from build123d import *

# Parameters (mm, degrees)
SKETCH1_W                                           = 60
SKETCH1_H                                           = 35
BOSS_EXTRUDE1_DEPTH                                 = 3
BOSS_EXTRUDE2_DEPTH                                 = 60
CUT_EXTRUDE4_DEPTH                                  = 49.961719741
CUT_EXTRUDE4_DEPTH_BACK                             = 49.961719741
SKETCH9_W                                           = 15
SKETCH9_H                                           = 12
CSK_FOR_M3_COUNTERSUNK_FLAT_HEAD_SCREW1_D           = 3.4
CSK_FOR_M3_COUNTERSUNK_FLAT_HEAD_SCREW1_DEPTH       = 3
CSK_FOR_M3_COUNTERSUNK_FLAT_HEAD_SCREW1_CSINK_D     = 6.3
CSK_FOR_M3_COUNTERSUNK_FLAT_HEAD_SCREW1_CSINK_ANGLE = 90
CSK_FOR_M3_COUNTERSUNK_FLAT_HEAD_SCREW1_TIP         = 1.021463052


with BuildPart() as part:
    # Sketch1 → Boss-Extrude1 (new body)
    with BuildSketch(Plane.XY):
        Rectangle(SKETCH1_W, SKETCH1_H)
    extrude(amount=BOSS_EXTRUDE1_DEPTH)

    # Sketch5 → Boss-Extrude2 (add)
    with BuildSketch(Plane(origin=(30, 0, 0), x_dir=(0, 0, -1), z_dir=(1, 0, 0))):
        with BuildLine():
            Line((-5.479055467, 14.545576741), (-4.958110934, 11.591153482))
            ThreePointArc((-4.958110934, 11.591153482), (-8.05212086, 23.138155725), (-3, 12.303847577))
            Line((-3, 12.303847577), (-3, 17.5))
            ThreePointArc((-3, 17.5), (-8.298133329, 19.428362829), (-5.479055467, 14.545576741))
        make_face()
    extrude(amount=-BOSS_EXTRUDE2_DEPTH)

    # Sketch9 → Cut-Extrude4 (cut, two sides: drawn at the far end of the back side and taken through both)
    with BuildSketch(Plane(origin=(-12, 0, 3), x_dir=(-1, 0, 0), z_dir=(0, 0, -1)).offset(-CUT_EXTRUDE4_DEPTH_BACK)):
        with Locations((-19.5, 17.5)):
            Rectangle(SKETCH9_W, SKETCH9_H)
        with Locations((10.5, 17.5)):
            Rectangle(SKETCH9_W, SKETCH9_H)
    extrude(amount=CUT_EXTRUDE4_DEPTH + CUT_EXTRUDE4_DEPTH_BACK, mode=Mode.SUBTRACT)

    # CSK for M3 Countersunk Flat Head Screw1
    with Locations(Plane(origin=(0, 0, 0), x_dir=(1, 0, 0), z_dir=(0, 0, -1))):
        with Locations((0, -4.5), (-15, 9.5), (15, 9.5)):
            CounterSinkHole(CSK_FOR_M3_COUNTERSUNK_FLAT_HEAD_SCREW1_D / 2, CSK_FOR_M3_COUNTERSUNK_FLAT_HEAD_SCREW1_CSINK_D / 2, depth=CSK_FOR_M3_COUNTERSUNK_FLAT_HEAD_SCREW1_DEPTH, counter_sink_angle=CSK_FOR_M3_COUNTERSUNK_FLAT_HEAD_SCREW1_CSINK_ANGLE)
            with Locations((0, 0, -(CSK_FOR_M3_COUNTERSUNK_FLAT_HEAD_SCREW1_DEPTH + CSK_FOR_M3_COUNTERSUNK_FLAT_HEAD_SCREW1_TIP / 2))):  # 118° drill point
                Cone(0, CSK_FOR_M3_COUNTERSUNK_FLAT_HEAD_SCREW1_D / 2, CSK_FOR_M3_COUNTERSUNK_FLAT_HEAD_SCREW1_TIP, mode=Mode.SUBTRACT)


solid = part.part
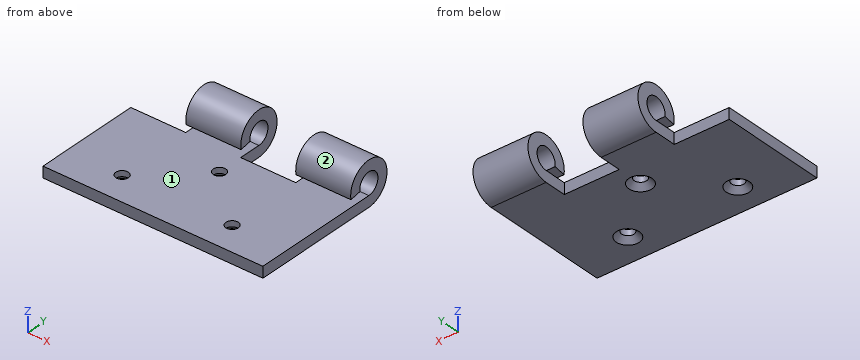
Work out the finished part from the listing and answer in its coordinate system (mm). Face numbers are marked on the shaded views. A direction names the side the tool comes from. Coordinates: 2 decimals unless noted, no trailing zeros. Order: outer loops, then holes, each group sorted by start corner. A loop starts at its lowest first (then second) coordinate and runs counter-clockwise, first axis right, second up. Notation, with made-up numbers: (24.5, 52) - (62.5, 52) arc R9 ccw to (62.5, 63) - close; hole circle Ø8 at (22, -35.75). An arc over 180 degrees is marked (long way). Put each result on its own line as item: value. Start each with the question number.
1) Find section A-A (y = 4.5). Give the vertices of the cut face in (x, z).
2) Find the intervals of material crossed by line 1 (X direction, y = 12, z = 6); line 2 (Z direction, x = -25.5, y = -14); line 3 (Z direction, x = 27, y = 15), in increasing order. Write a range as from..to.
3) Find section B-B (z = 4). Give the vertices of the cut face in (x, y).
4) For the marked faces 1 and 2, determine the directions among +Z, -Z, +X, -X, +Y, -Y from which every point of the face is accessible in a straight line to the end or side of a thin tool.
5) Find section D-D (z = 10.25). Give the vertices of the cut face in (x, y), plus the area to 3 significant figures.
6) Flat-ended cylindrical pins translate along their axes: pin 1 (5 mm diameter, centred on x = -11.5, y = 14.5, fed in from +Z); pin 2 (2 mm diameter, centred on x = -12, y = 14, fed in from -Z); pin 3 (4.5 mm diameter, centred on x = -15, y = -9.5, fed in from -Z); pin 4 (1.5 mm diameter, centred on x = 8.5, z = 1.5, fed in from +Y). Find the tip coordinate at first contact, or state that the pin passes through.
7) Find section C-C (x = -4.5). Give the vertices of the cut face in (y, z).
Results list:
1. outline: (-30, 0) - (-3.15, 0) - (-1.7, 1.45) - (-1.7, 3) - (-30, 3) - close; (1.7, 1.45) - (3.15, 0) - (30, 0) - (30, 3) - (1.7, 3) - close
2. line 1: x = -15..0, 15..30
2. line 2: z = 0..3
2. line 3: z = 0..3, 7.66..11.45
3. outline: (-15, 19.74) - (0, 19.74) - (0, 23.16) - (-15, 23.16) - close; (15, 19.74) - (30, 19.74) - (30, 23.16) - (15, 23.16) - close
4. face 1: +X, -X, -Y
4. face 2: +X, -X
5. outline: (-15, 13.26) - (0, 13.26) - (0, 21.74) - (-15, 21.74) - close; (15, 13.26) - (30, 13.26) - (30, 21.74) - (15, 21.74) - close
5. area: 254 mm^2
6. pin 1: stops at z = 11.98
6. pin 2: stops at z = 0
6. pin 3: stops at z = 0.9
6. pin 4: stops at y = 11.5
7. outline: (-17.5, 0) - (17.5, 0) arc R6 ccw (long way) to (11.59, 4.96) - (14.55, 5.48) arc R3 cw (long way) to (17.5, 3) - (-17.5, 3) - close
